Can you work these out from the model? Positions are in its coordinate system, mm. A direction names the side the tool comes from. Round coordinates to 2 decimals unless told otherwise and drop trailing zeros. Order: outer loops, then holes, each group sorted by start corner. A loop starts at its lowest first (then second) coordinate and runs counter-clockwise, first axis right, second up. Notation, with made-up numbers: (63.25, -39) -> (89.25, -39) arc R5 cw to (89.25, -31) -> close; hole circle Ø10 at (-11, -32). An arc over 180 degrees is marked (long way). Use a Markdown table: item, result. Add a question column.
Q1. If we section it at B-B on x = -2.75: List the corners of the cut face in (y, z) for me, plus the area to 3 significant figures.
Q2. We'd pull the mould along Y, two halves only. Please class faces 4 (the face through (0, 90, 7)), 5 (the face through (0, 82, 10)), 6 (the face through (0, 65, 10)), 7 (the face through (0, 74, 7)): +Y half, -Y half, draft (parallel to the pull), parting line (faces both ways), or undercut.
Q3. If we section it at D-D on z = 14.5: List the corners of the cut face in (x, y) for me.
Q4. I need wall thicknesses on line 1 along Z through (x, y) = (-0.5, 81.25); line 2 along X through (y, z) = (73.75, 2.75); line 3 along Z through (x, y) = (0, 87.75). Which ranges of each line are inside material? Lowest first, please. Write a range as [from, to].
Q5. If we section it at C-C on y = 82: List the corners of the cut face in (x, z) for me, plus the area to 3 significant figures.
Q6. If we section it at A-A on z = 7.5: List the corners of the cut face in (x, y) for me, plus the area to 3 significant figures.
Q7. For faces 1 (the face through (-0.1, 73.6, 3.5)), 2 (the face through (-7.27, 74.48, 6.8)), 3 (the face through (7.305, 74.51, 6.796)), which set-ups out of +Z, -Z, +X, -X, +Y, -Y let a thin tool reach every point of the face, with its end or its side?
Q8. I'm going to push flat-ended pins straight in: pin 1 Ø2 at (x, z) = (-3, 7.5) entering from -Y; pin 2 Ø8 at (x, y) = (8.5, 79) entering from +Z; pin 3 Ø3 at (y, z) = (80, 4.5) entering from +X. Where does each tip first touch, or does it pass through?
```python
from build123d import *

# Parameters (mm, degrees)
BOSS_EXTRUDE1_DEPTH = 20
CUT_EXTRUDE1_START  = -3.5
CUT_EXTRUDE1_DEPTH  = 3.5
CUT_EXTRUDE2_START  = -16.5
CUT_EXTRUDE2_DEPTH  = 16.5
CUT_EXTRUDE3_START  = -10
CUT_EXTRUDE3_DEPTH  = 10
BOSS_EXTRUDE2_START = -3.5
BOSS_EXTRUDE2_DEPTH = 3.5
FILLET1_R           = 2


with BuildPart() as part:
    # Sketch1 → Boss-Extrude1 (new body)
    with BuildSketch(Plane.XY):
        with BuildLine():
            Line((-8.978202217, 83.518811563), (-7.7250269, 74))
            ThreePointArc((-7.7250269, 74), (-8.71901412, 73.889477149), (-9.711425926, 73.765603414))
            Line((-9.711425926, 73.765603414), (-8.484202494, 64.443915989))
            ThreePointArc((-8.484202494, 64.443915989), (0, 65), (8.484202494, 64.443915989))
            Line((8.484202494, 64.443915989), (9.711425926, 73.765603414))
            ThreePointArc((9.711425926, 73.765603414), (8.71901412, 73.889477149), (7.7250269, 74))
            Line((7.7250269, 74), (8.978202217, 83.518811563))
            Line((8.978202217, 83.518811563), (9.761566637, 89.469055079))
            ThreePointArc((9.761566637, 89.469055079), (0, 90), (-9.761566637, 89.469055079))
            Line((-9.761566637, 89.469055079), (-8.978202217, 83.518811563))
        make_face()
    extrude(amount=BOSS_EXTRUDE1_DEPTH)

    # Sketch2 → Cut-Extrude1 (cut)
    with BuildSketch(Plane(origin=(0, 0, 0), x_dir=(-1, 0, 0), z_dir=(0, 0, -1)).offset(CUT_EXTRUDE1_START)):
        with BuildLine():
            Line((-9.761566637, 89.469055079), (-8.978202217, 83.518811563))
            ThreePointArc((-8.978202217, 83.518811563), (0, 84), (8.978202217, 83.518811563))
            Line((8.978202217, 83.518811563), (9.761566637, 89.469055079))
            ThreePointArc((9.761566637, 89.469055079), (0, 90), (-9.761566637, 89.469055079))
        make_face()
    extrude(amount=CUT_EXTRUDE1_DEPTH, mode=Mode.SUBTRACT)

    # Sketch3 → Cut-Extrude2 (cut)
    with BuildSketch(Plane.XY.offset(20).offset(CUT_EXTRUDE2_START)):
        with BuildLine():
            Line((7.7250269, 74), (-7.7250269, 74))
            ThreePointArc((-7.7250269, 74), (-8.71901412, 73.889477149), (-9.711425926, 73.765603414))
            Line((-9.711425926, 73.765603414), (-9.267359648, 70.392585158))
            ThreePointArc((-9.267359648, 70.392585158), (0, 71), (9.267359648, 70.392585158))
            Line((9.267359648, 70.392585158), (9.711425926, 73.765603414))
            ThreePointArc((9.711425926, 73.765603414), (8.71901412, 73.889477149), (7.7250269, 74))
        make_face()
    extrude(amount=CUT_EXTRUDE2_DEPTH, mode=Mode.SUBTRACT)

    # Sketch4 → Cut-Extrude3 (cut)
    with BuildSketch(Plane.XY.offset(20).offset(CUT_EXTRUDE3_START)):
        with BuildLine():
            Line((-7.7250269, 74), (7.7250269, 74))
            Line((7.7250269, 74), (9.761566637, 89.469055079))
            ThreePointArc((9.761566637, 89.469055079), (0, 90), (-9.761566637, 89.469055079))
            Line((-9.761566637, 89.469055079), (-7.7250269, 74))
        make_face()
    extrude(amount=CUT_EXTRUDE3_DEPTH, mode=Mode.SUBTRACT)

    # Sketch5 → Boss-Extrude2 (add)
    with BuildSketch(Plane.XY.offset(3.5).offset(BOSS_EXTRUDE2_START)):
        with BuildLine():
            Line((9.711425926, 73.765603414), (10.964200146, 83.281368355))
            ThreePointArc((10.964200146, 83.281368355), (9.971907933, 83.406001296), (8.978202217, 83.518811563))
            Line((8.978202217, 83.518811563), (7.7250269, 74))
            ThreePointArc((7.7250269, 74), (8.71901412, 73.889477149), (9.711425926, 73.765603414))
        make_face()
        with BuildLine():
            Line((-9.711425926, 73.765603414), (-10.964200146, 83.281368355))
            ThreePointArc((-10.964200146, 83.281368355), (-9.971907933, 83.406001296), (-8.978202217, 83.518811563))
            Line((-8.978202217, 83.518811563), (-7.7250269, 74))
            ThreePointArc((-7.7250269, 74), (-8.71901412, 73.889477149), (-9.711425926, 73.765603414))
        make_face()
    extrude(amount=BOSS_EXTRUDE2_DEPTH)

    # Fillet1
    fillet1_edges = [part.edges().sort_by_distance(p)[0] for p in [
        (7.7250269, 74, 6.75),
        (-7.7250269, 74, 6.75),
        (9.761566637, 89.469055079, 6.75),
        (-9.761566637, 89.469055079, 6.75),
    ]]
    fillet(fillet1_edges, radius=FILLET1_R)


solid = part.part
```
Answer below:
| question | item | result |
|---|---|---|
| 1 | outline | (64.94, 0) -> (83.95, 0) -> (83.95, 3.5) -> (89.96, 3.5) -> (89.96, 10) -> (74, 10) -> (74, 3.5) -> (70.95, 3.5) -> (70.95, 20) -> (64.94, 20) -> close |
| 1 | area | 269 mm² |
| 2 | face 4 | +Y half |
| 2 | face 5 | draft |
| 2 | face 6 | -Y half |
| 2 | face 7 | undercut |
| 3 | outline | (-9.27, 70.39) -> (-8.48, 64.44) arc R65 cw to (8.48, 64.44) -> (9.27, 70.39) arc R71 ccw to start |
| 4 | line 1 | [0, 10] |
| 4 | line 2 | [-9.71, 9.71] |
| 4 | line 3 | [3.5, 10] |
| 5 | outline | (-10.8, 0) -> (10.8, 0) -> (10.8, 3.5) -> (8.78, 3.5) -> (8.78, 10) -> (-8.78, 10) -> (-8.78, 3.5) -> (-10.8, 3.5) -> close |
| 5 | area | 190 mm² |
| 6 | outline | (-9.49, 87.42) -> (-7.95, 75.74) arc R2 ccw to (-5.97, 74) -> (5.97, 74) arc R2 ccw to (7.95, 75.74) -> (9.49, 87.42) arc R2 ccw to (7.68, 89.67) arc R90 ccw to (-7.68, 89.67) arc R2 ccw to start; (-9.27, 70.39) -> (-8.48, 64.44) arc R65 cw to (8.48, 64.44) -> (9.27, 70.39) arc R71 ccw to start |
| 6 | area | 381 mm² |
| 7 | face 1 | +Z |
| 7 | face 2 | +Z, -X |
| 7 | face 3 | +Z, +X |
| 8 | pin 1 | y = 64.88 |
| 8 | pin 2 | z = 10 |
| 8 | pin 3 | x = 10.68 |
